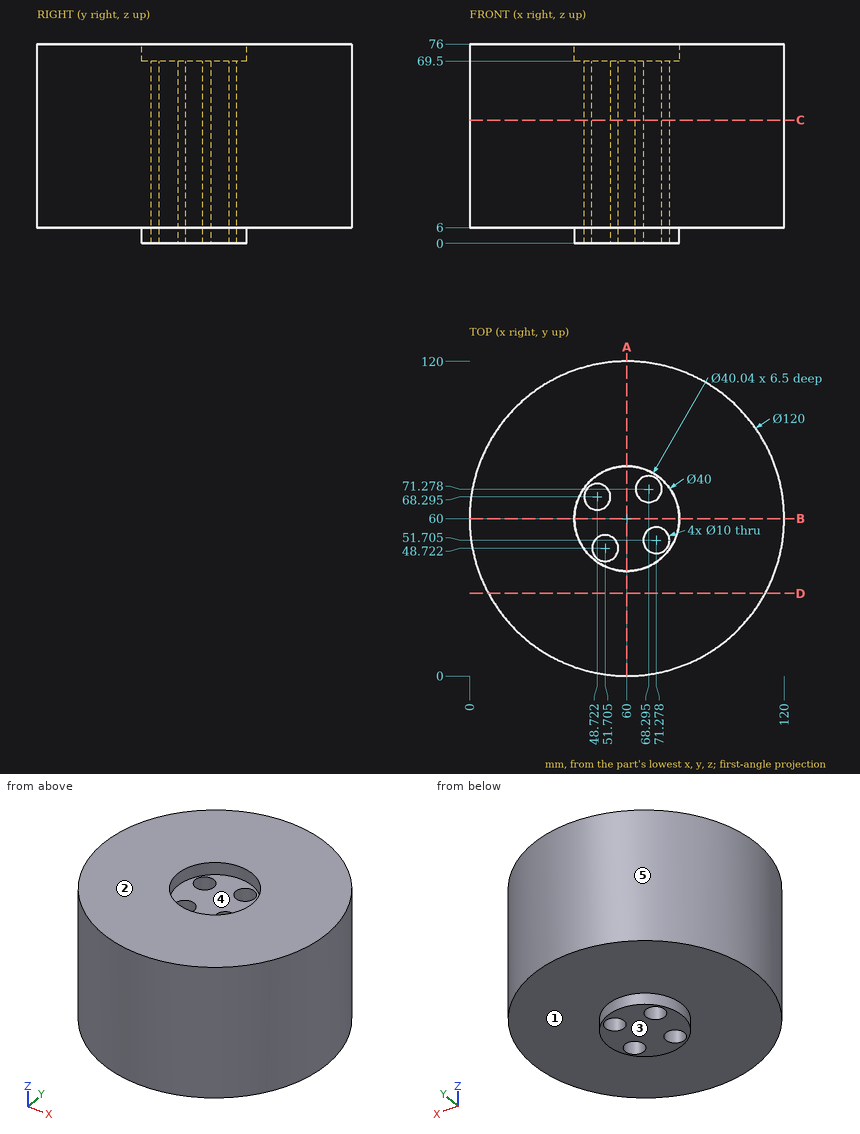
For this review, use the dimensioned drawing (mm, ordinates from the lowest corner) and the shaded views. A direction names the side the tool comes from. Round coordinates to 2 decimals unless told otherwise and drop trailing zeros. Write each loop counter-clockwise with the first axis right and the second up, starting at its lowest first coordinate (ties: lowest second). Pieces come first, ordered by that corner, then holes. Notation, with made-up numbers: (83, 65.25) -> (93, 65.25) arc R19 ccw to (93, 84.25) -> close; hole circle Ø2 at (13.25, 1.25). An arc over 180 degrees is marked (long way). Use one line per item in the form item = value.
Q1. Clearance check with flat-ended pins moving along their axes: pin 1 Ø12 at (x, y) = (52.5, 61) entering from +Z; pin 2 Ø1 at (y, z) = (26.5, 9.5) entering from +X; pin 3 Ø10 at (x, z) = (23.5, 64) entering from -Y (1 decimal). State where each tip first meets the part, or that it passes through.
Resolved:
pin_1 = 69.5
pin_2 = 110.11
pin_3 = 8.9
Q2. To check wall thickness, follow probe 1 along Z at (x, y) = (42, 99); probe 2 along X at (y, z) = (69.5, 58.5) (1 decimal); probe 3 along Y at (x, z) = (71, 73.5) (1 decimal). State the ranges of each line that lie inside material, in increasing order. Write a range as from..to.
Resolved:
probe_1 = 6..76
probe_2 = 0.8..43.9, 53.6..63.6, 73..119.2
probe_3 = 1..43.3, 76.7..119
Q3. The part is to be moulded in two halves that separate along Y. For the marked faces 3, 4 and 5, say which applies: released by +Y, released by -Y, zero draft, split by the parting line, or undercut.
Resolved:
face_3 = zero draft
face_4 = undercut
face_5 = split by the parting line
Q4. Consider section D-D (y = 31.5). State the section outline as (x, z) points.
Resolved:
outline = (7.2, 6) -> (112.8, 6) -> (112.8, 76) -> (7.2, 76) -> close
Q5. Consider section C-C (z = 47). State the section outline as (x, y) points (1 decimal), then the cut area to 3 significant figures.
Resolved:
outline = circle Ø120 at (60, 60); hole circle Ø10 at (48.7, 68.3); hole circle Ø10 at (51.7, 48.7); hole circle Ø10 at (68.3, 71.3); hole circle Ø10 at (71.3, 51.7)
area = 11,000 mm²
Q6. Machinability: for the marked faces 1 and 2, which of the approach directions +Z, -Z, +X, -X, +Y, -Y give a long, thin tool a straight path to every point of the face, cutting with its end or side? Answer none if there is none.
Resolved:
face_1 = -Z
face_2 = +Z, +X, -X, +Y, -Y
Q7. Consider section A-A (x = 60). State the section outline as (y, z) points, then the cut area to 3 significant figures.
Resolved:
outline = (0, 6) -> (40, 6) -> (40, 0) -> (80, 0) -> (80, 6) -> (120, 6) -> (120, 76) -> (80.02, 76) -> (80.02, 69.5) -> (39.98, 69.5) -> (39.98, 76) -> (0, 76) -> close
area = 8,380 mm²
